Design review of the part built by this model. Coordinates are the model's own, in mm. A direction names the side the tool comes from. Round coordinates to 2 decimals unless told otherwise and drop trailing zeros. Write each loop counter-clockwise with the first axis right and the second up, starting at its lowest first coordinate (ties: lowest second). Pieces come first, ordered by that corner, then holes.
from build123d import *

# Parameters (mm, degrees)
CROQUIS1_W              = 280
CROQUIS1_H              = 162
CROQUIS1_W_2            = 270
CROQUIS1_H_2            = 152
SALIENTE_EXTRUIR1_DEPTH = 45
CROQUIS3_W              = 280
CROQUIS3_H              = 162
SALIENTE_EXTRUIR2_DEPTH = 4
CROQUIS4_W              = 5
CROQUIS4_H              = 152
SALIENTE_EXTRUIR3_DEPTH = 45


with BuildPart() as part:
    # Croquis1 → Saliente-Extruir1 (new body)
    with BuildSketch(Plane(origin=(0, 0, 0), x_dir=(1, 0, 0), z_dir=(0, 1, 0))):
        Rectangle(CROQUIS1_W, CROQUIS1_H)
        Rectangle(CROQUIS1_W_2, CROQUIS1_H_2, mode=Mode.SUBTRACT)
    extrude(amount=SALIENTE_EXTRUIR1_DEPTH)

    # Croquis3 → Saliente-Extruir2 (add)
    with BuildSketch(Plane.XZ):
        Rectangle(CROQUIS3_W, CROQUIS3_H)
    extrude(amount=SALIENTE_EXTRUIR2_DEPTH)

    # Croquis4 → Saliente-Extruir3 (add)
    with BuildSketch(Plane(origin=(0, 0, 0), x_dir=(1, 0, 0), z_dir=(0, 1, 0))):
        with Locations((52.5, 0)):
            Rectangle(CROQUIS4_W, CROQUIS4_H)
    extrude(amount=SALIENTE_EXTRUIR3_DEPTH)


solid = part.part
1) For line 1 along X through (y, z) = (19, 26.5); line 2 along Z through (x, y) = (-114, 37); line 3 along Y through (x, z) = (44, 74), list the stretches that pass through material, from the lowest coordinate up.
2) Add section A-A on y = 11. State the section outline as (x, z) points.
3) The part is to be moulded in two halves that separate along X. For faces 3 (the face through (-140, 21, -1)), 4 (the face through (-2, 21, 81)), 5 (the face through (-44, 22, -76)), say which applies: pulls with the +X half, pulls with the -X half, needs draft (parallel to the pull), parting line crosses it, or undercut.
4) For faces 1 (the face through (-2, -4, 1)), 2 (the face through (94, 22, 76)), list the 3-axis set-ups (+Z, -Z, +X, -X, +Y, -Y) from which the entire face can be reached by the end or side of a thin tool; tool diameter is ignored.
5) Add section C-C on x = -53.5. State the section outline as (y, z) points.
6) Add section B-B on z = -55.5. State the section outline as (x, y) points.
7) For P1, Ø1.5, axis at x = 80, z = -37.5, coming from the +Y side, flat-tipped, find the tip position at first contact; note if it passes through.
Computed:
1. line 1: x = -140 to -135, 50 to 55, 135 to 140
1. line 2: z = -81 to -76, 76 to 81
1. line 3: y = -4 to 0
2. outline: (-140, -81) - (140, -81) - (140, 81) - (-140, 81) - close; hole (-135, -76) - (50, -76) - (50, 76) - (-135, 76) - close; hole (55, -76) - (135, -76) - (135, 76) - (55, 76) - close
3. face 3: pulls with the -X half
3. face 4: needs draft
3. face 5: undercut
4. face 1: +Z, -Z, +X, -X, -Y
4. face 2: +Y
5. outline: (-4, -81) - (45, -81) - (45, -76) - (0, -76) - (0, 76) - (45, 76) - (45, 81) - (-4, 81) - close
6. outline: (-140, -4) - (140, -4) - (140, 45) - (135, 45) - (135, 0) - (55, 0) - (55, 45) - (50, 45) - (50, 0) - (-135, 0) - (-135, 45) - (-140, 45) - close
7. P1: stops at y = 0
